Geometry: see drawing. Coordinates: mm, zero at the bounding-box minimum. A direction names the side the tool comes from. Round coordinates to 2 decimals unless told otherwise and drop trailing zeros. Write each loop counter-clockwise with the first axis right and the second up, starting at its lowest first coordinate (ties: lowest second). Pieces come first, ordered by that corner, then holes. Notation, with made-up numbers: M -35.5,-9.5 L 5.5,-9.5 A23 ccw 5.5,27.5 Z; hole C -22,79.5 d9. An arc over 180 degrees is marked long. Use one line per item in the form item = value. Start each with the question number.
Item 1: Section query A-A (x = 120). Return loops of the section in (y, z).
Item 2: Section query D-D (z = 153). Return loops of the section in (x, y).
Item 3: Section query C-C (y = 29). Return loops of the section in (x, z), and give its area (3 significant figures).
Item 4: Ray query, probe 1 along X at (y, z) = (57, 120); probe 2 along Y at (x, z) = (27, 180); probe 3 along X at (y, z) = (35.5, 207.5). Return the intervals inside material, ascending.
Item 5: Reachability of the marked faces 1 and 2 from +Z, -Z, +X, -X, +Y, -Y: full face, straight path, thin tool, end or side. Return the list, or none.
Item 6: Pin query (flat end, axial travel): pin 1 Ø10 at (y, z) = (37, 194.5) entering from +X; pin 2 Ø8 at (x, y) = (138.5, 49.5) entering from +Z; pin 3 Ø1.5 at (x, y) = (112, 40) entering from -Z. Return the tip coordinate at first contact, or that it passes through.
Item 7: Section query B-B (z = 120). Return loops of the section in (x, y), and give its area (3 significant figures).
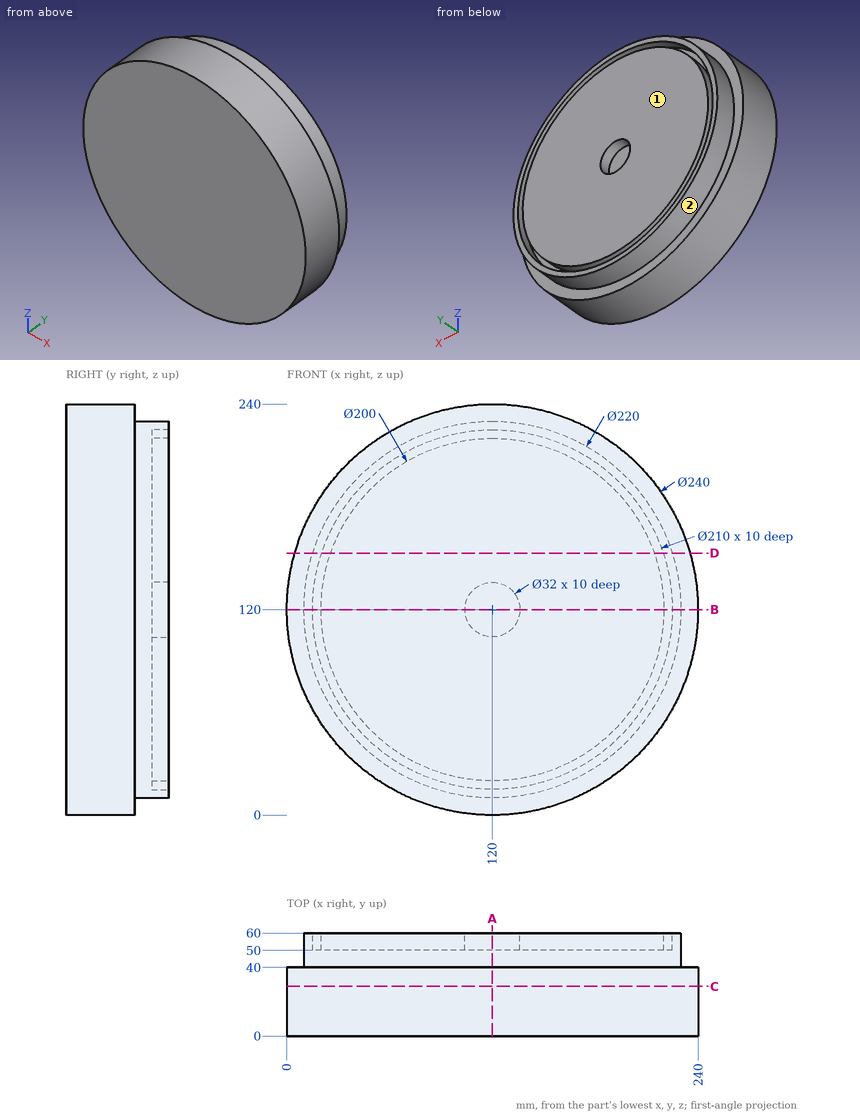
Working result:
q1.outline = M 0,0 L 40,0 L 40,10 L 60,10 L 60,15 L 50,15 L 50,20 L 60,20 L 60,104 L 50,104 L 50,136 L 60,136 L 60,220 L 50,220 L 50,225 L 60,225 L 60,230 L 40,230 L 40,240 L 0,240 Z
q2.outline = M 4.63,0 L 235.37,0 L 235.37,40 L 224.93,40 L 224.93,60 L 219.68,60 L 219.68,50 L 214.4,50 L 214.4,60 L 25.6,60 L 25.6,50 L 20.32,50 L 20.32,60 L 15.07,60 L 15.07,40 L 4.63,40 Z
q3.outline = C 120,120 d240
q3.area = 45,200 mm²
q4.probe_1 = 10 to 15, 20 to 104, 136 to 220, 225 to 230
q4.probe_2 = 0 to 40
q4.probe_3 = 37.88 to 202.12
q5.face_1 = +Z, -Z, +X, -X, +Y
q5.face_2 = +Y
q6.pin_1 = 217.83
q6.pin_2 = 229.04
q6.pin_3 = 0.22
q7.outline = M 0,0 L 240,0 L 240,40 L 230,40 L 230,60 L 225,60 L 225,50 L 220,50 L 220,60 L 136,60 L 136,50 L 104,50 L 104,60 L 20,60 L 20,50 L 15,50 L 15,60 L 10,60 L 10,40 L 0,40 Z
q7.area = 13,600 mm²
